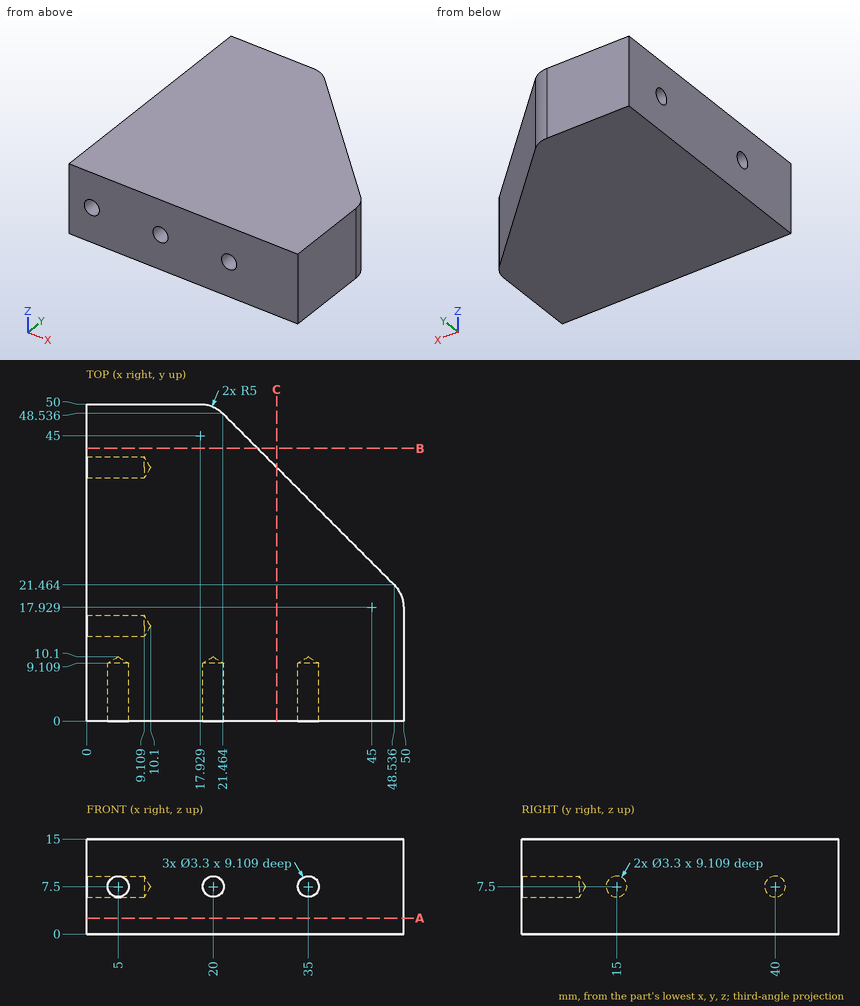
Answer from the drawing. Dimensions are ordinates in mm from the lowest x, y and z of the part. Round coordinates to 2 decimals unless told otherwise and drop trailing zeros. Write each loop counter-clockwise with the first axis right and the second up, starting at its lowest first coordinate (ties: lowest second). Pieces come first, ordered by that corner, then holes.
1. Straight lines are drawn through the part: L1, parallel to X at y = 7, z = 7.5; L2, parallel to Y at x = 7.25, z = 7.5; L3, parallel to Z at x = 4, y = 40. For each, find the intervals that lie inside material, in ascending order.
2. The part is cut by section A-A, the plane z = 2.5. Determine the outline of the cut face in (x, y) (1 decimal), then the cut area to 3 significant figures.
3. Given pin 1 Ø2.5 at (x, z) = (5, 7.5) entering from -Y; pin 2 Ø2 at (y, z) = (40, 7.5) entering from +X; pin 3 Ø1 at (y, z) = (32.5, 4.5) entering from +X, each flat-ended and moving along its own axis, determine where each tip first touches the part or whether it passes through.
4. The part is cut by section B-B, the plane y = 43. Determine the outline of the cut face in (x, z).
5. The part is cut by section C-C, the plane x = 30. Determine the outline of the cut face in (y, z).
Values:
1. L1: x = 0 to 3.35, 6.65 to 18.35, 21.65 to 33.35, 36.65 to 50
1. L2: y = 0 to 13.35, 16.65 to 38.35, 41.65 to 50
1. L3: z = 0 to 5.85, 9.15 to 15
2. outline: (0, 0) - (50, 0) - (50, 17.9) arc R5 ccw to (48.5, 21.5) - (21.5, 48.5) arc R5 ccw to (17.9, 50) - (0, 50) - close
2. area: 2,050 mm2
3. pin 1: stops at y = 9.35
3. pin 2: stops at x = 31
3. pin 3: stops at x = 38
4. outline: (0, 0) - (27, 0) - (27, 15) - (0, 15) - close
5. outline: (0, 0) - (40, 0) - (40, 15) - (0, 15) - close
